Part model, mm, in its own coordinate system. Give positions to 0.01 mm unless a question says otherwise; leave off trailing zeros. Write each loop counter-clockwise with the first axis right and the second up, starting at its lowest first coordinate (ties: lowest second). Pieces come first, ordered by that corner, then holes. Notation, with made-up numbers: M 77,13 L 109,13 A11 ccw 109,18 Z; hole C 77,81 d9. An arc over 180 degrees is marked long. Answer as CSV lines item,"result". Start each with the question number.
1) Wall check: line 1 along Y through (x, z) = (11.25, 144); line 2 along Y through (x, z) = (11.5, 142); line 3 along Z through (x, y) = (1, 71). Give the ranges that are in metal, low to high. Write a range as from..to.
2) Pin check, flat tips, straight feed: pin 1 Ø2 at (x, z) = (9, 172.5) entering from -Y; pin 2 Ø6 at (x, z) = (3.5, 57) entering from +Y; pin 3 Ø3 at (x, z) = (1.5, 110) entering from -Y. Stop position of each tip, or through.
3) Slice it at A-A, the plane x = 4.75. Give the cut face in (y, z).
4) Slice it at C-C, the plane z = 57. Give the cut face in (x, y), plus the area to 3 significant figures.
5) Slice it at B-B, the plane y = -186. Give the cut face in (x, z).
```python
from build123d import *

# Parameters (mm, degrees)
F1_DEPTH = 12.7


with BuildPart() as f1:
    # F0 (on Right) → F1 (new body)
    with BuildSketch(Plane.YZ):
        with BuildLine():
            ThreePointArc((-68.898448, 178.096197), (-74.992037, 177.056382), (-80.653981, 174.575369))
            ThreePointArc((-80.653981, 174.575369), (-208.301311, 92.096861), (-329.192638, 0))
            Line((-329.192638, 0), (-319.189282, 0))
            ThreePointArc((-319.189282, 0), (-201.534739, 89.085299), (-77.506695, 169.059209))
            Line((-77.506695, 169.059209), (-73.337511, 171.530273))
            Line((-73.337511, 171.530273), (356.607362, 191.762973))
            Line((356.607362, 191.762973), (356.607362, 198.12))
            Line((356.607362, 198.12), (-68.898448, 178.096197))
        make_face()
    extrude(amount=F1_DEPTH)


solid = f1.part
```
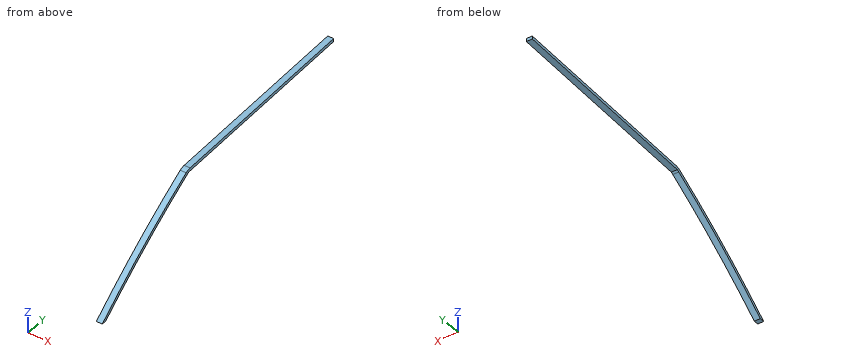
Found:
1,line 1,"-130.54..-118.63"
1,line 2,"-133.69..-121.81"
1,line 3,"178.32..184.68"
2,pin 1,"y = -85.83"
2,pin 2,"y = -242.01"
2,pin 3,"y = -184.58"
3,outline,"M -329.19,0 L -319.19,0 A1958.65 cw -77.51,169.06 L -73.34,171.53 L 356.61,191.76 L 356.61,198.12 L -68.9,178.1 A25.4 ccw -80.65,174.58 A1965 ccw Z"
4,outline,"M 0,-256.69 L 12.7,-256.69 L 12.7,-246.06 L 0,-246.06 Z"
4,area,"135 mm²"
5,outline,"M 0,99.84 L 12.7,99.84 L 12.7,107.53 L 0,107.53 Z"
